```python
from build123d import *

# Parameters (mm, degrees)
BOSS_EXTRUDE1_DEPTH = 6
CUT_EXTRUDE1_REACH  = 35.779
BOSS_EXTRUDE2_DEPTH = 30
CUT_EXTRUDE2_REACH  = 50.374
SKETCH5_R           = 2
CUT_EXTRUDE3_DEPTH  = 50
CHAMFER1_SIZE       = 10.392304845
CHAMFER1_SIZE_2     = 6
CHAMFER2_SIZE       = 10.392304845
CHAMFER2_SIZE_2     = 6
CUT_EXTRUDE4_DEPTH  = 4


with BuildPart() as part:
    # Sketch1 → Boss-Extrude1 (new body)
    with BuildSketch(Plane.XY):
        with BuildLine():
            Line((-25, 0), (0, 0))
            Line((0, 0), (25, 0))
            Line((25, 0), (25, -12))
            Line((25, -12), (-25, -12))
            ThreePointArc((-25, -12), (-31, -6), (-25, 0))
        make_face()
    extrude(amount=BOSS_EXTRUDE1_DEPTH)

    # Sketch2 → Cut-Extrude1 (cut, up to next)
    with BuildSketch(Plane.XY.offset(6), mode=Mode.PRIVATE) as cut_extrude1_sk1:
        with BuildLine():
            Line((-28.05, -6), (-21.95, -6))
            ThreePointArc((-21.95, -6), (-25, -2.95), (-28.05, -6))
        make_face()
    cut_extrude1_tool1 = extrude(cut_extrude1_sk1.sketch, amount=-CUT_EXTRUDE1_REACH, mode=Mode.PRIVATE) & part.part
    add(cut_extrude1_tool1.solids().sort_by_distance((-25, -4.70554, 6))[0], mode=Mode.SUBTRACT)

    # Sketch3 → Boss-Extrude2 (add)
    with BuildSketch(Plane(origin=(0, 0, 0), x_dir=(-1, 0, 0), z_dir=(0, 0, -1))):
        Polygon((-25, 0), (-5, 0), (-5, -6), (-5, -12), (-25, -12), align=None)
    extrude(amount=BOSS_EXTRUDE2_DEPTH)

    # Sketch4 → Cut-Extrude2 (cut, up to next)
    with BuildSketch(Plane.ZY.offset(-5), mode=Mode.PRIVATE) as cut_extrude2_sk1:
        Polygon((-20.968911087, -6), (-24, -4.25), (-24, -7.75), align=None)
    cut_extrude2_tool1 = extrude(cut_extrude2_sk1.sketch, amount=-CUT_EXTRUDE2_REACH, mode=Mode.PRIVATE) & part.part
    add(cut_extrude2_tool1.solids().sort_by_distance((5, -6, -22.989637))[0], mode=Mode.SUBTRACT)

    # Sketch5 → Cut-Extrude3 (cut, through all)
    with BuildSketch(Plane.XY.offset(6)):
        with Locations((15, -6)):
            Circle(SKETCH5_R)
    extrude(amount=-CUT_EXTRUDE3_DEPTH, mode=Mode.SUBTRACT)

    # Chamfer1
    # the kernel refuses this chamfer: 10.392304845, 6 mm, written as the material it takes off along each edge
    with BuildSketch(Plane(origin=(5, 0, 0), x_dir=(0.9998132206222079, 0.019326765612700622, 0), z_dir=(0, 0, -1))) as chamfer1_piece_1:
        Polygon((CHAMFER1_SIZE * 0.999813220662, CHAMFER1_SIZE * 0.0193267656135), (-CHAMFER1_SIZE_2 * 0.0193267656127, CHAMFER1_SIZE_2 * 0.999813220622), (0, 0), align=None)
    extrude(amount=56.885783824, mode=Mode.SUBTRACT)
    with BuildSketch(Plane(origin=(5, -12, 0), x_dir=(-0.057893862402671484, 0.9983227437537926, 0), z_dir=(0, 0, -1))) as chamfer1_piece_2:
        Polygon((CHAMFER1_SIZE_2 * 0.998322743754, CHAMFER1_SIZE_2 * 0.0578938624027), (-CHAMFER1_SIZE * 0.057893862405, CHAMFER1_SIZE * 0.998322743793), (0, 0), align=None)
    extrude(amount=56.885783824, mode=Mode.SUBTRACT)

    # Chamfer2
    # the kernel refuses this chamfer: 10.392304845, 6 mm, written as the material it takes off along each edge
    with BuildSketch(Plane(origin=(25, -12, 32.885783824), x_dir=(-0.9998132206222079, -0.01932676561270069, 0), z_dir=(0, 0, -1))) as chamfer2_piece_1:
        Polygon((CHAMFER2_SIZE * 0.999813220662, CHAMFER2_SIZE * 0.0193267656135), (-CHAMFER2_SIZE_2 * 0.0193267656127, CHAMFER2_SIZE_2 * 0.999813220622), (0, 0), align=None)
    extrude(amount=89.771567647, mode=Mode.SUBTRACT)
    with BuildSketch(Plane(origin=(25, 0, 32.885783824), x_dir=(-0.9998132206222079, 0.019326765612700622, 0), z_dir=(0, 0, -1))) as chamfer2_piece_2:
        Polygon((CHAMFER2_SIZE * 0.999813220662, -CHAMFER2_SIZE * 0.0193267656135), (-CHAMFER2_SIZE_2 * 0.0193267656127, -CHAMFER2_SIZE_2 * 0.999813220622), (0, 0), align=None)
    extrude(amount=89.771567647, mode=Mode.SUBTRACT)

    # Sketch6 → Cut-Extrude4 (cut)
    with BuildSketch(Plane.XY.offset(-30)):
        Polygon((11.4, -3.921539031), (11.4, -8.078460969), (15, -10.156921938), (18.6, -8.078460969), (18.6, -3.921539031), (15, -1.843078062), align=None)
    extrude(amount=CUT_EXTRUDE4_DEPTH, mode=Mode.SUBTRACT)


solid = part.part
```
CAD build for the part. Positions are in the model's coordinates, mm. A direction names the side the tool comes from. Coordinates: 2 decimals unless noted, no trailing zeros. Loops run counter-clockwise (first coordinate to the right, second up) from the corner with the lowest first, then second, coordinate; pieces in that order, holes last. Notation, with made-up numbers: (83, -14) - (88, -14) arc R20 cw to (88, -6) - close; hole circle Ø11 at (-31, 41). An arc over 180 degrees is marked (long way). Use CSV: the item, a comma, the result in double quotes. Start each with the question number.
Q1. 3-axis set-ups, long thin cutter, end or side, ignore diameter. For faces 5 (the flat face through (-5, -12, 3)), 6 (the flat face through (17, -9, -28)), 7 (the flat face through (9.93, -8.846, -14.79)), 8 (the flat face through (10.07, -3.073, -14.79)), 9 (the cylindrical face through (-31, -6, 3)): which of +Z, -Z, +X, -X, +Y, -Y reach the whole face in a straight line?
Q2. Cut at B-B, the plane x = 19.5. List the corners of the cut face in (y, z), then the cut area to 3 significant figures.
Q3. Cut at D-D, the plane x = -19. List the corners of the cut face in (y, z), then the cut area to 3 significant figures.
Q4. Two-plate mould, pull along Z, no slides. Class faces 1 (the flat face through (11, -6, -30)), 2 (the flat face through (-25, -6, 3)), 3 (the flat face through (20.42, -6.89, -22.51)), 4 (the flat face through (9, -6, -24)): +Z half, -Z half, draft (parallel to the pull), parting line (faces both ways), or undercut.
Q5. Cut at C-C, the plane z = -13. List the corners of the cut face in (x, y), then the cut area to 3 significant figures.
Q6. Drop flat-ended pins along their axis: P1, Ø1, axis at x = -23.5, y = -4, coming from the -Z side; P2, Ø6.5, axis at x = 15, y = -6, coming from the -Z side; P3, Ø4, axis at y = -10.5, z = -26.5, coming from the -X side; P4, Ø2, axis at y = -6, z = -27, coming from the -X side. Give the stop position or say it passes through.
Q7. Cut at A-A, the plane y = -5. List the corners of the cut face in (x, z), then the cut area to 3 significant figures.
Q8. Probe probe 1 along Y at (x, z) = (15, -5.5); probe 2 along Z at (x, y) = (1.5, -10); probe 3 along X at (y, z) = (-7, -5). List the from-to ranges inside material, lowest first. Write a range as from..to.
Here are the results:
1,face 5,"+Z, -Z, +X, -X, -Y"
1,face 6,"-Z"
1,face 7,"-Z, -X, -Y"
1,face 8,"-Z, -X, +Y"
1,face 9,"+Z, -Z, -X"
2,outline,"(-9.18, -30) - (-2.82, -30) - (-2.82, 6) - (-9.18, 6) - close; hole (-7.75, -24) - (-4.25, -24) - (-6, -20.97) - close"
2,area,"223 mm2"
3,outline,"(-12, 0) - (0, 0) - (0, 6) - (-12, 6) - close"
3,area,"72.0 mm2"
4,face 1,"-Z half"
4,face 2,"draft"
4,face 3,"undercut"
4,face 4,"undercut"
5,outline,"(5, -6) - (15, -11.77) - (25, -6) - (15, -0.23) - close; hole circle Ø4 at (15, -6)"
5,area,"103 mm2"
6,P1,"through"
6,P2,"z = -26"
6,P3,"x = 9.33"
6,P4,"x = 5"
7,outline,"(-30.92, 0) - (-27.88, 0) - (-27.88, 6) - (-30.92, 6) - close; (-22.12, 0) - (6.73, 0) - (6.73, -22.7) - (13.27, -22.7) - (13.27, 6) - (-22.12, 6) - close; (6.73, -30) - (11.4, -30) - (11.4, -26) - (13.27, -26) - (13.27, -24) - (6.73, -24) - close; (16.73, -26) - (18.6, -26) - (18.6, -30) - (23.27, -30) - (23.27, -24) - (16.73, -24) - close; (16.73, -22.7) - (23.27, -22.7) - (23.27, 6) - (16.73, 6) - close"
7,area,"630 mm2"
8,probe 1,"-11.77..-8, -4..-0.23"
8,probe 2,"0..6"
8,probe 3,"6.73..13.27, 16.73..23.27"
